For this review, take the finished solid that the model builds, in its own axes (mm). Round coordinates to 2 decimals unless told otherwise and drop trailing zeros. Loops run counter-clockwise (first coordinate to the right, second up) from the corner with the lowest first, then second, coordinate; pieces in that order, holes last.
1) Insertion check: pin 1 (19 mm diameter, centred on x = 14, z = -26.5, fed in from -Y). The pin has a flat end and moves straight along its axis. Give the tip position at first contact, or say it passes through.
2) Take a section at B-B (y = 1.5). State the section outline as (x, z) points.
3) Take a section at C-C (x = 12.5). State the section outline as (y, z) points, then the cut area to 3 significant figures.
4) Take a section at A-A (x = 0). State the section outline as (y, z) points.
5) Wall thickness on L1, parallel to Y at x = 29, z = -39; L2, parallel to Y at x = 1, z = -38.5; L3, parallel to X at y = 1.75, z = -52: over which ranges is each line inside the solid? List them lowest first.
```python
from build123d import *

# Parameters (mm, degrees)
F0_W      = 63.608665
F0_H      = 99.548988
F2_DEPTH  = 7.95075
F3_R      = 5.08
F4_R      = 5.08
F5_R      = 5.08
F6_R      = 5.08
F8_W      = 63.608665
F8_H      = 99.548988
F8_R      = 1.663226
F8_W_2    = 51.913798
F8_H_2    = 77.585458
F9_DEPTH  = 2.95953
F1_W      = 51.913798
F1_H      = 77.585458
F10_DEPTH = 2.82358


with BuildPart() as f2:
    # F0 (on Front) → F2 (new body)
    with BuildSketch(Plane.XZ):
        with Locations((-0.14262, -7.416256)):
            Rectangle(F0_W, F0_H)
    extrude(amount=-F2_DEPTH)

    # F3
    f3_edges = [f2.edges().sort_by_distance(p)[0] for p in [
        (-31.946953, 3.975375, 42.358238),
    ]]
    fillet(f3_edges, radius=F3_R)

    # F4
    f4_edges = [f2.edges().sort_by_distance(p)[0] for p in [
        (31.661712, 3.975375, 42.358238),
    ]]
    fillet(f4_edges, radius=F4_R)

    # F5
    f5_edges = [f2.edges().sort_by_distance(p)[0] for p in [
        (31.661712, 3.975375, -57.19075),
    ]]
    fillet(f5_edges, radius=F5_R)

    # F6
    f6_edges = [f2.edges().sort_by_distance(p)[0] for p in [
        (-31.946953, 3.975375, -57.19075),
    ]]
    fillet(f6_edges, radius=F6_R)

    # F8 (on face) → F9 (cut)
    with BuildSketch(Plane.XZ):
        with Locations((-0.14262, -7.416256)):
            Rectangle(F8_W, F8_H)
        with Locations((0, -52.056417)):
            Circle(F8_R, mode=Mode.SUBTRACT)
        with Locations((0, -6.703157)):
            Rectangle(F8_W_2, F8_H_2, mode=Mode.SUBTRACT)
    extrude(amount=-F9_DEPTH, mode=Mode.SUBTRACT)

    # F1 (on face) → F10 (cut)
    with BuildSketch(Plane.XZ):
        with Locations((0, -6.703157)):
            Rectangle(F1_W, F1_H)
    extrude(amount=-F10_DEPTH, mode=Mode.SUBTRACT)


solid = f2.part
```
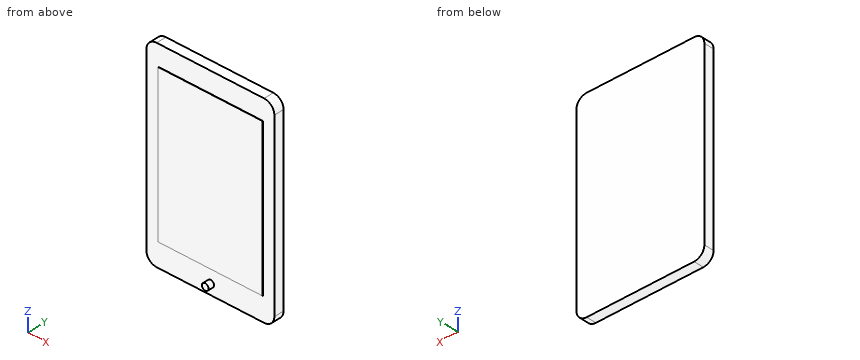
Response:
1. pin 1: stops at y = 2.82
2. outline: circle Ø3.33 at (0, -52.06)
3. outline: (2.82, -45.5) - (2.96, -45.5) - (2.96, -57.19) - (7.95, -57.19) - (7.95, 42.36) - (2.96, 42.36) - (2.96, 32.09) - (2.82, 32.09) - close
3. area: 507 mm2
4. outline: (0, -53.72) - (2.96, -53.72) - (2.96, -57.19) - (7.95, -57.19) - (7.95, 42.36) - (2.96, 42.36) - (2.96, 32.09) - (2.82, 32.09) - (2.82, -45.5) - (2.96, -45.5) - (2.96, -50.39) - (0, -50.39) - close
5. L1: y = 2.96 to 7.95
5. L2: y = 2.82 to 7.95
5. L3: x = -1.66 to 1.66
